Answer from the drawing. Dimensions are ordinates in mm from the lowest x, y and z of the part. A direction names the side the tool comes from. Give positions to 0.01 mm unless a question says otherwise; leave off trailing zeros. Order: outer loops, then holes, each group sorted by start corner. A loop starts at its lowest first (then second) coordinate and runs counter-clockwise, first axis right, second up. Notation, with made-up numbers: (58, 59.5) - (97, 59.5) arc R20 ccw to (97, 80.5) - close; hole circle Ø2 at (88.5, -8.75). An arc over 180 degrees is marked (long way). Answer in a Markdown table with one row per item. Add a question column.
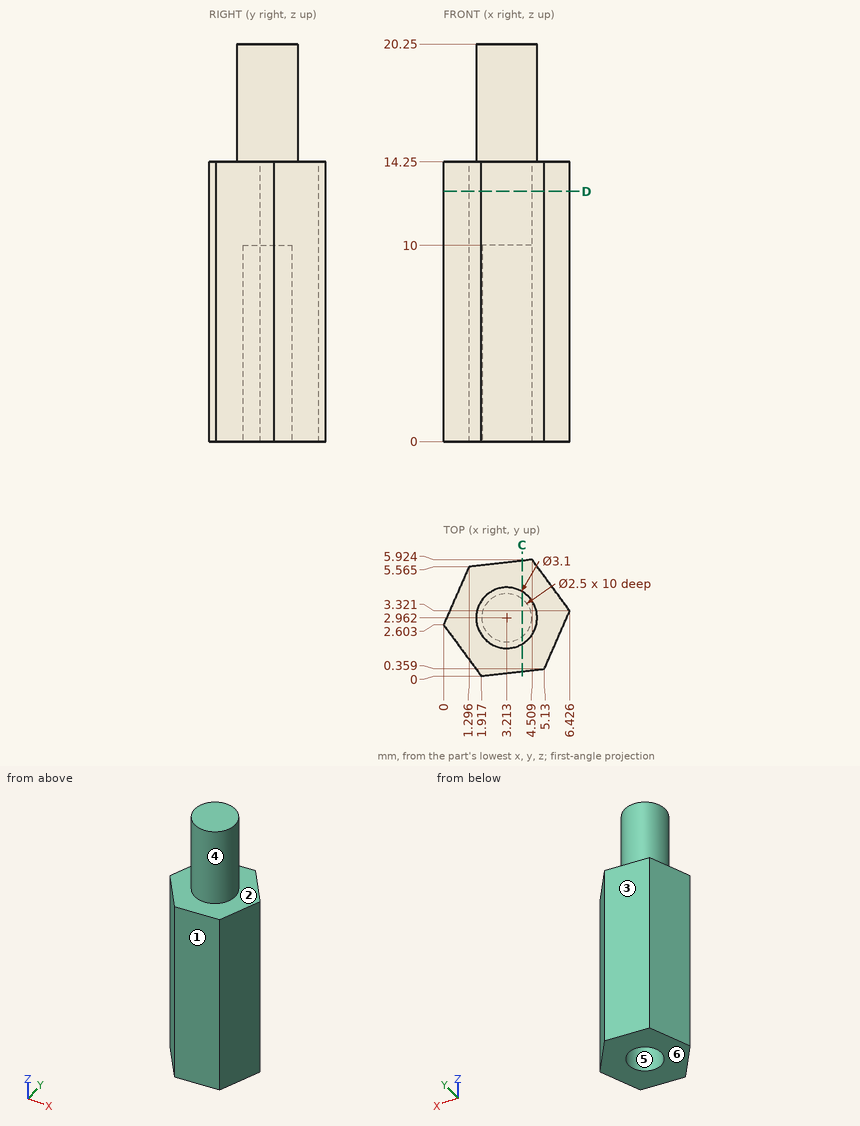
(1) The mould has two halves that part along X. Classify the marked faces 3, 4, 5 and 6: +X half, -X half, draft (parallel to the pull), parting line (faces both ways), or undercut.
(2) Each of these flat-tipped pins is pushed along its axis until it touches: P1, Ø1.2, axis at x = 3, y = 3, coming from the -Z side; P2, Ø1, axis at y = 3, z = 18, coming from the -X side; P3, Ø1.5, axis at y = 1, z = 18, coming from the +X side. Where does it stop, or does it pass through?
(3) Straight lines are drawn through the part: line 1 (Z direction, x = 2.25, y = 4.8); line 2 (Z direction, x = 3.25, y = 2); line 3 (X direction, y = 2.05, z = 8.25) (1 decimal). For each, find the intervals that lie inside material, in ascending order.
(4) Find section C-C, the plane x = 4. Write down the section's boundary in (y, z).
(5) For the marked faces 1 and 2, determine the directions among +Z, -Z, +X, -X, +Y, -Y from which every point of the face is accessible in a straight line to the end or side of a thin tool.
(6) Find section D-D, the plane z = 12.75. Write down the section's boundary in (x, y) (1 decimal).
Answer key:
| question | item | result |
|---|---|---|
| 1 | face 3 | -X half |
| 1 | face 4 | parting line |
| 1 | face 5 | undercut |
| 1 | face 6 | draft |
| 2 | P1 | z = 10 |
| 2 | P2 | x = 1.66 |
| 2 | P3 | x = 4.18 |
| 3 | line 1 | 0 to 14.25 |
| 3 | line 2 | 10 to 20.25 |
| 3 | line 3 | 0.4 to 2.4, 4.1 to 5.9 |
| 4 | outline | (0.23, 0) - (1.99, 0) - (1.99, 10) - (3.93, 10) - (3.93, 0) - (5.87, 0) - (5.87, 14.25) - (4.3, 14.25) - (4.3, 20.25) - (1.63, 20.25) - (1.63, 14.25) - (0.23, 14.25) - close |
| 5 | face 1 | +Z, -Z, +X, -Y |
| 5 | face 2 | +Z |
| 6 | outline | (0, 2.6) - (1.9, 0) - (5.1, 0.4) - (6.4, 3.3) - (4.5, 5.9) - (1.3, 5.6) - close |
